from build123d import *

# Parameters (mm, degrees)
SKETCH1_R                = 3.5
BOSS_EXTRUDE1_DEPTH      = 3
BOSS_EXTRUDE1_DEPTH_BACK = 9
BOSS_EXTRUDE2_DEPTH      = 3
BOSS_EXTRUDE3_DEPTH      = 1.9


with BuildPart() as part:
    # Sketch1 → Boss-Extrude1 (new body, two sides)
    with BuildSketch(Plane.ZY.offset(-64.468173267)) as boss_extrude1_sk:
        with Locations((260.861627804, 7.55)):
            Circle(SKETCH1_R)
    extrude(amount=BOSS_EXTRUDE1_DEPTH)
    extrude(boss_extrude1_sk.sketch, amount=-BOSS_EXTRUDE1_DEPTH_BACK)

    # Sketch2 → Boss-Extrude2 (add)
    with BuildSketch(Plane.ZY.offset(-61.468173267)):
        Polygon((263.418922822, 3.130759561), (265.967449799, 7.555062231), (263.410154781, 11.974302669), (258.304332787, 11.969240439), (255.75580581, 7.544937769), (258.313100828, 3.125697331), align=None)
    extrude(amount=-BOSS_EXTRUDE2_DEPTH)

    # Sketch3 → Boss-Extrude3 (add)
    with BuildSketch(Plane(origin=(73.468173267, 0, 0), x_dir=(0, 0, -1), z_dir=(1, 0, 0))):
        Polygon((-258.313100828, 3.125697331), (-255.75580581, 7.544937769), (-258.304332787, 11.969240439), (-263.410154781, 11.974302669), (-265.967449799, 7.555062231), (-263.418922822, 3.130759561), align=None)
    extrude(amount=BOSS_EXTRUDE3_DEPTH)


solid = part.part
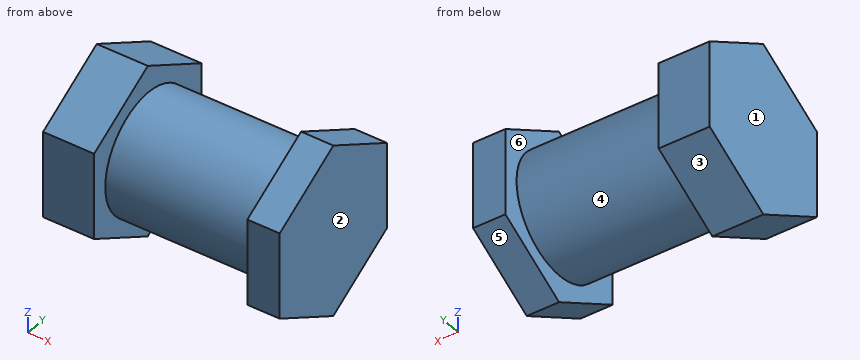
Can you work these out from the model? Positions are in its coordinate system, mm. Face numbers are marked on the shaded views. A direction names the side the tool comes from. Give positions to 0.01 mm unless a question says otherwise; leave off trailing zeros. Order: outer loops, then holes, each group sorted by start corner. A loop starts at its lowest first (then second) coordinate and runs counter-clockwise, first axis right, second up. Notation, with made-up numbers: M 36,-4 L 44,-4 A27 cw 44,28 Z; hole C -28.5,52.25 d7. An arc over 180 degrees is marked long. Use one line per item in the form item = value. Start each with the question number.
Item 1: We'd pull the mould along X, two halves only. Please class the marked faces 1, 2, 3 and 4: +X half, -X half, draft (parallel to the pull), parting line (faces both ways), or undercut.
Item 2: For the marked faces 5 and 6, which set-ups out of +Z, -Z, +X, -X, +Y, -Y let a thin tool reach every point of the face, with its end or its side?
Item 3: Will these pins go through, and if not, where does the flat tip stop? pin 1 Ø1.5 at (x, y) = (72.5, 9.5) entering from -Z; pin 2 Ø1.5 at (x, y) = (66, 6.5) entering from -Z; pin 3 Ø1.5 at (x, y) = (66, 10) entering from -Z.
Item 4: If we section it at D-D (y = 4.75): Write out the boundary of the cut face in (x, z), then the cut area to 3 significant figures.
Item 5: If I drill on line 1 along X through (y, z) = (11.25, 258.25); line 2 along Y through (x, z) = (70, 261); line 3 along Y through (x, z) = (68.5, 263.5), over which ranges is the centre line in solid material (lowest first)?
Item 6: If we section it at C-C (x = 70.5): Write out the boundary of the cut face in (y, z).
Item 7: If we section it at B-B (z = 262.5): Write out the boundary of the cut face in (x, y).
Item 8: If we section it at A-A (z = 256.5): Write out the boundary of the cut face in (x, y).
Outcome:
q1.face_1 = -X half
q1.face_2 = +X half
q1.face_3 = draft
q1.face_4 = undercut
q2.face_5 = -Z, +X, -X, +Y
q2.face_6 = none
q3.pin_1 = 257.57
q3.pin_2 = 257.37
q3.pin_3 = 257.8
q4.outline = M 61.47,257.37 L 64.47,257.37 L 64.47,258.76 L 73.47,258.76 L 73.47,257.37 L 75.37,257.37 L 75.37,264.35 L 73.47,264.35 L 73.47,262.96 L 64.47,262.96 L 64.47,264.35 L 61.47,264.35 Z
q4.area = 72.0 mm2
q5.line_1 = 61.47 to 64.47, 73.47 to 75.37
q5.line_2 = 4.05 to 11.05
q5.line_3 = 5.25 to 9.85
q6.outline = C 7.55,260.86 d7
q7.outline = M 61.47,3.13 L 64.47,3.13 L 64.47,4.46 L 73.47,4.46 L 73.47,3.13 L 75.37,3.13 L 75.37,11.97 L 73.47,11.97 L 73.47,10.64 L 64.47,10.64 L 64.47,11.97 L 61.47,11.97 Z
q8.outline = M 61.47,6.26 L 64.47,6.26 L 64.47,8.84 L 61.47,8.84 Z; M 73.47,6.26 L 75.37,6.26 L 75.37,8.84 L 73.47,8.84 Z
